from build123d import *

# Parameters (mm, degrees)
BOSS_EXTRU_1_DEPTH      = 1
ESQUISSE2_W             = 63.121311346
ESQUISSE2_H             = 43.227445896
ENL_V_MAT_EXTRU_1_DEPTH = 1
ENL_V_MAT_EXTRU_2_DEPTH = 1
ESQUISSE4_R             = 1.25
ENL_V_MAT_EXTRU_3_DEPTH = 1


with BuildPart() as part:
    # Esquisse1 → Boss.-Extru.1 (new body)
    with BuildSketch(Plane.XY):
        with BuildLine():
            Line((-32.05, -59.71), (32.05, -59.71))
            ThreePointArc((32.05, -59.71), (34.185462479, -58.825462479), (35.07, -56.69))
            Line((35.07, -56.69), (35.07, 56.69))
            ThreePointArc((35.07, 56.69), (34.185462479, 58.825462479), (32.05, 59.71))
            Line((32.05, 59.71), (-32.05, 59.71))
            ThreePointArc((-32.05, 59.71), (-34.185462479, 58.825462479), (-35.07, 56.69))
            Line((-35.07, 56.69), (-35.07, -56.69))
            ThreePointArc((-35.07, -56.69), (-34.185462479, -58.825462479), (-32.05, -59.71))
        make_face()
    extrude(amount=BOSS_EXTRU_1_DEPTH)

    # Esquisse2 → Enlèv. mat.-Extru.1 (cut)
    with BuildSketch(Plane.XY.offset(1)):
        with Locations((-0.068131464, 36.133663017)):
            Rectangle(ESQUISSE2_W, ESQUISSE2_H)
    extrude(amount=-ENL_V_MAT_EXTRU_1_DEPTH, mode=Mode.SUBTRACT)

    # Esquisse3 → Enlèv. mat.-Extru.2 (cut)
    with BuildSketch(Plane.XY.offset(1)):
        with BuildLine():
            Line((-5.450287773, -54.403229927), (12.482160985, -54.403229927))
            ThreePointArc((12.482160985, -54.403229927), (13.189267766, -54.110336708), (13.482160985, -53.403229927))
            Line((13.482160985, -53.403229927), (13.482160985, -49.311147183))
            ThreePointArc((13.482160985, -49.311147183), (13.775054203, -48.604040402), (14.482160985, -48.311147183))
            Line((14.482160985, -48.311147183), (18.639313678, -48.311147183))
            ThreePointArc((18.639313678, -48.311147183), (19.346420459, -48.604040402), (19.639313678, -49.311147183))
            Line((19.639313678, -49.311147183), (19.639313678, -53.403229927))
            ThreePointArc((19.639313678, -53.403229927), (19.932206896, -54.110336708), (20.639313678, -54.403229927))
            Line((20.639313678, -54.403229927), (31.226680359, -54.403229927))
            ThreePointArc((31.226680359, -54.403229927), (31.93378714, -54.110336708), (32.226680359, -53.403229927))
            Line((32.226680359, -53.403229927), (32.226680359, -12.723689117))
            ThreePointArc((32.226680359, -12.723689117), (31.93378714, -12.016582336), (31.226680359, -11.723689117))
            Line((31.226680359, -11.723689117), (-30.58163263, -11.723689117))
            ThreePointArc((-30.58163263, -11.723689117), (-31.288739411, -12.016582336), (-31.58163263, -12.723689117))
            Line((-31.58163263, -12.723689117), (-31.58163263, -53.403229927))
            ThreePointArc((-31.58163263, -53.403229927), (-31.288739411, -54.110336708), (-30.58163263, -54.403229927))
            Line((-30.58163263, -54.403229927), (-13.536578839, -54.403229927))
            ThreePointArc((-13.536578839, -54.403229927), (-12.829472057, -54.110336708), (-12.536578839, -53.403229927))
            Line((-12.536578839, -53.403229927), (-12.536578839, -49.311147183))
            ThreePointArc((-12.536578839, -49.311147183), (-12.24368562, -48.604040402), (-11.536578839, -48.311147183))
            Line((-11.536578839, -48.311147183), (-7.450287773, -48.311147183))
            ThreePointArc((-7.450287773, -48.311147183), (-6.743180992, -48.604040402), (-6.450287773, -49.311147183))
            Line((-6.450287773, -49.311147183), (-6.450287773, -53.403229927))
            ThreePointArc((-6.450287773, -53.403229927), (-6.157394554, -54.110336708), (-5.450287773, -54.403229927))
        make_face()
        with BuildLine():
            Line((-14.910409974, 2.342410274), (-9.548047777, 2.342410274))
            ThreePointArc((-9.548047777, 2.342410274), (-8.840940996, 2.049517055), (-8.548047777, 1.342410274))
            Line((-8.548047777, 1.342410274), (-8.548047777, -2.145402138))
            ThreePointArc((-8.548047777, -2.145402138), (-8.840940996, -2.85250892), (-9.548047777, -3.145402138))
            Line((-9.548047777, -3.145402138), (-14.910409974, -3.145402138))
            ThreePointArc((-14.910409974, -3.145402138), (-15.617516755, -3.438295357), (-15.910409974, -4.145402138))
            Line((-15.910409974, -4.145402138), (-15.910409974, -7.633214551))
            ThreePointArc((-15.910409974, -7.633214551), (-16.203303193, -8.340321332), (-16.910409974, -8.633214551))
            Line((-16.910409974, -8.633214551), (-19.922709244, -8.633214551))
            ThreePointArc((-19.922709244, -8.633214551), (-20.629816025, -8.340321332), (-20.922709244, -7.633214551))
            Line((-20.922709244, -7.633214551), (-20.922709244, -4.145402138))
            ThreePointArc((-20.922709244, -4.145402138), (-21.215602463, -3.438295357), (-21.922709244, -3.145402138))
            Line((-21.922709244, -3.145402138), (-27.434575926, -3.145402138))
            ThreePointArc((-27.434575926, -3.145402138), (-28.141682707, -2.85250892), (-28.434575926, -2.145402138))
            Line((-28.434575926, -2.145402138), (-28.434575926, 1.342410274))
            ThreePointArc((-28.434575926, 1.342410274), (-28.141682707, 2.049517055), (-27.434575926, 2.342410274))
            Line((-27.434575926, 2.342410274), (-21.922709244, 2.342410274))
            ThreePointArc((-21.922709244, 2.342410274), (-21.215602463, 2.635303493), (-20.922709244, 3.342410274))
            Line((-20.922709244, 3.342410274), (-20.922709244, 6.336052927))
            ThreePointArc((-20.922709244, 6.336052927), (-20.629816025, 7.043159708), (-19.922709244, 7.336052927))
            Line((-19.922709244, 7.336052927), (-16.910409974, 7.336052927))
            ThreePointArc((-16.910409974, 7.336052927), (-16.203303193, 7.043159708), (-15.910409974, 6.336052927))
            Line((-15.910409974, 6.336052927), (-15.910409974, 3.342410274))
            ThreePointArc((-15.910409974, 3.342410274), (-15.617516755, 2.635303493), (-14.910409974, 2.342410274))
        make_face()
        with BuildLine():
            Line((22.256339951, 2.342410274), (28.131649076, 2.342410274))
            ThreePointArc((28.131649076, 2.342410274), (28.838755857, 2.049517055), (29.131649076, 1.342410274))
            Line((29.131649076, 1.342410274), (29.131649076, -2.145402138))
            ThreePointArc((29.131649076, -2.145402138), (28.838755857, -2.85250892), (28.131649076, -3.145402138))
            Line((28.131649076, -3.145402138), (22.256339951, -3.145402138))
            ThreePointArc((22.256339951, -3.145402138), (21.54923317, -3.438295357), (21.256339951, -4.145402138))
            Line((21.256339951, -4.145402138), (21.256339951, -7.633214551))
            ThreePointArc((21.256339951, -7.633214551), (20.963446732, -8.340321332), (20.256339951, -8.633214551))
            Line((20.256339951, -8.633214551), (17.869767116, -8.633214551))
            ThreePointArc((17.869767116, -8.633214551), (17.162660335, -8.340321332), (16.869767116, -7.633214551))
            Line((16.869767116, -7.633214551), (16.869767116, -4.145402138))
            ThreePointArc((16.869767116, -4.145402138), (16.576873898, -3.438295357), (15.869767116, -3.145402138))
            Line((15.869767116, -3.145402138), (10.124858061, -3.145402138))
            ThreePointArc((10.124858061, -3.145402138), (9.41775128, -2.85250892), (9.124858061, -2.145402138))
            Line((9.124858061, -2.145402138), (9.124858061, 1.342410274))
            ThreePointArc((9.124858061, 1.342410274), (9.41775128, 2.049517055), (10.124858061, 2.342410274))
            Line((10.124858061, 2.342410274), (15.869767116, 2.342410274))
            ThreePointArc((15.869767116, 2.342410274), (16.576873898, 2.635303493), (16.869767116, 3.342410274))
            Line((16.869767116, 3.342410274), (16.869767116, 6.336052927))
            ThreePointArc((16.869767116, 6.336052927), (17.162660335, 7.043159708), (17.869767116, 7.336052927))
            Line((17.869767116, 7.336052927), (20.256339951, 7.336052927))
            ThreePointArc((20.256339951, 7.336052927), (20.963446732, 7.043159708), (21.256339951, 6.336052927))
            Line((21.256339951, 6.336052927), (21.256339951, 3.342410274))
            ThreePointArc((21.256339951, 3.342410274), (21.54923317, 2.635303493), (22.256339951, 2.342410274))
        make_face()
        with BuildLine():
            Line((11.114053306, 12.655752766), (14.294222496, 12.655752766))
            ThreePointArc((14.294222496, 12.655752766), (15.001329278, 12.362859547), (15.294222496, 11.655752766))
            Line((15.294222496, 11.655752766), (15.294222496, 7.930302608))
            ThreePointArc((15.294222496, 7.930302608), (15.001329278, 7.223195827), (14.294222496, 6.930302608))
            Line((14.294222496, 6.930302608), (11.114053306, 6.930302608))
            ThreePointArc((11.114053306, 6.930302608), (10.406946525, 7.223195827), (10.114053306, 7.930302608))
            Line((10.114053306, 7.930302608), (10.114053306, 11.655752766))
            ThreePointArc((10.114053306, 11.655752766), (10.406946525, 12.362859547), (11.114053306, 12.655752766))
        make_face()
    extrude(amount=-ENL_V_MAT_EXTRU_2_DEPTH, mode=Mode.SUBTRACT)

    # Esquisse4 → Enlèv. mat.-Extru.3 (cut)
    with BuildSketch(Plane.XY.offset(1)):
        with Locations((-30.226, -6.858)):
            Circle(ESQUISSE4_R)
        with Locations((29.845, -9.017)):
            Circle(ESQUISSE4_R)
        with Locations((16.51, -51.562)):
            Circle(ESQUISSE4_R)
        with Locations((-10.16, -51.562)):
            Circle(ESQUISSE4_R)
    extrude(amount=-ENL_V_MAT_EXTRU_3_DEPTH, mode=Mode.SUBTRACT)


solid = part.part
Geometry: final body of the model. Coordinates: model frame, mm. Round coordinates to 2 decimals unless told otherwise and drop trailing zeros. Loops run counter-clockwise (first coordinate to the right, second up) from the corner with the lowest first, then second, coordinate; pieces in that order, holes last.
Q1. Pull-direction query (Y, two-part tool) for faces 1 (the flat face through (0, 5, 0)), 2 (the cylindrical face through (34.16, -58.85, 0.49)), 3 (the cylindrical face through (-10.323, -50.323, 0.507)), 4 (the cylindrical face through (16.347, -50.323, 0.507)); classes: released by +Y, released by -Y, zero draft, split by the parting line, or undercut.
Q2. Section A-A on x = 24. Return loops of the section in (y, z).
Q3. Section D-D on z = 0.6. State how many separate pieces and enclosed holes the cut face has, plus the area to 3 significant figures.
Q4. Section B-B on y = 49.5. Return loops of the section in (x, z).
Q5. Section C-C on x = 8. Return loops of the section in (y, z), plus the area to 3 significant figures.
Q6. Material intervals for L1, parallel to X at y = 4, z = 0.45; L2, parallel to Y at x = 11.5, z = 0.6; L3, parallel to Y at x = -5, z = 0.15, sorted ascending.
Evaluation:
1. face 1: zero draft
1. face 2: released by -Y
1. face 3: undercut
1. face 4: undercut
2. outline: (-59.71, 0) - (-54.4, 0) - (-54.4, 1) - (-59.71, 1) - close; (-11.72, 0) - (-3.15, 0) - (-3.15, 1) - (-11.72, 1) - close; (2.34, 0) - (14.52, 0) - (14.52, 1) - (2.34, 1) - close; (57.75, 0) - (59.71, 0) - (59.71, 1) - (57.75, 1) - close
3. separate pieces: 1
3. enclosed holes: 9
3. area: 2,630 mm2
4. outline: (-35.07, 0) - (-31.63, 0) - (-31.63, 1) - (-35.07, 1) - close; (31.49, 0) - (35.07, 0) - (35.07, 1) - (31.49, 1) - close
5. outline: (-59.71, 0) - (-54.4, 0) - (-54.4, 1) - (-59.71, 1) - close; (-11.72, 0) - (14.52, 0) - (14.52, 1) - (-11.72, 1) - close; (57.75, 0) - (59.71, 0) - (59.71, 1) - (57.75, 1) - close
5. area: 33.5 mm2
6. L1: x = -35.07 to -20.92, -15.91 to 16.87, 21.26 to 35.07
6. L2: y = -59.71 to -54.4, -11.72 to -3.15, 2.34 to 6.93, 12.66 to 14.52, 57.75 to 59.71
6. L3: y = -59.71 to -54.4, -11.72 to 14.52, 57.75 to 59.71
